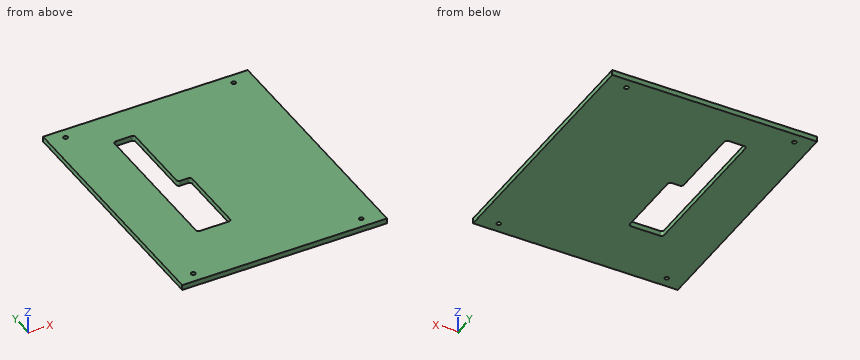
from build123d import *

# Parameters (mm, degrees)
ESQUISSE1_W        = 195
ESQUISSE1_H        = 240
ESQUISSE1_R        = 2.05
ESQUISSE1_W_2      = 32.5
ESQUISSE1_H_2      = 145
ESQUISSE1_W_3      = 12.5
ESQUISSE1_H_3      = 75
BOSS_EXTRU_1_DEPTH = 5
CONG_1_R           = 2.5


with BuildPart() as part:
    # Esquisse1 → Boss.-Extru.1 (new body)
    # profile 1 of 2: a face of its own
    with BuildSketch(Plane.XY):
        with Locations((-22.5, 0)):
            Rectangle(ESQUISSE1_W, ESQUISSE1_H)
        with Locations((56, -110)):
            Circle(ESQUISSE1_R, mode=Mode.SUBTRACT)
        with Locations((56, 110)):
            Circle(ESQUISSE1_R, mode=Mode.SUBTRACT)
        with Locations((-104, 110)):
            Circle(ESQUISSE1_R, mode=Mode.SUBTRACT)
        with Locations((-104, -110)):
            Circle(ESQUISSE1_R, mode=Mode.SUBTRACT)
        with Locations((-56.25, 12.5)):
            Rectangle(ESQUISSE1_W_2, ESQUISSE1_H_2, mode=Mode.SUBTRACT)
    # profile 2 of 2: a face of its own
    with BuildSketch(Plane.XY):
        with Locations((-46.25, 47.5)):
            Rectangle(ESQUISSE1_W_3, ESQUISSE1_H_3)
    extrude(amount=BOSS_EXTRU_1_DEPTH)

    # Congé1
    cong_1_edges = [part.edges().sort_by_distance(p)[0] for p in [
        (-72.5, 85, 2.5),
        (-72.5, -60, 2.5),
        (-40, -60, 2.5),
        (-40, 10, 2.5),
        (-52.5, 10, 2.5),
        (-52.5, 85, 2.5),
    ]]
    fillet(cong_1_edges, radius=CONG_1_R)


solid = part.part
Verification items for the finished model (mm, model axes). Coordinates: 2 decimals unless noted, no trailing zeros. Order: outer loops, then holes, each group sorted by start corner. A loop starts at its lowest first (then second) coordinate and runs counter-clockwise, first axis right, second up. Notation, with made-up numbers: M 70,15 L 80,15 A18 cw 80,21 Z; hole C -8,67.25 d1. An arc over 180 degrees is marked long. Write each question's results on one line, items separated by ' | '.
1) Section check B-B on z = 0.95. Record the cut outline in (x, y), plus the area to 3 significant figures.
Solved:
outline: M -120,-120 L 75,-120 L 75,120 L -120,120 Z; hole C -104,-110 d4.1; hole C -104,110 d4.1; hole M -72.5,-57.5 A2.5 ccw -70,-60 L -42.5,-60 A2.5 ccw -40,-57.5 L -40,7.5 A2.5 ccw -42.5,10 L -50,10 A2.5 cw -52.5,12.5 L -52.5,82.5 A2.5 ccw -55,85 L -70,85 A2.5 ccw -72.5,82.5 Z; hole C 56,-110 d4.1; hole C 56,110 d4.1 | area: 43,000 mm²
2) Section check A-A on y = 74.5. Record the cut outline in (x, z).
Solved:
outline: M -120,0 L -72.5,0 L -72.5,5 L -120,5 Z; M -52.5,0 L 75,0 L 75,5 L -52.5,5 Z
3) Scan lines: line 1 along Y through (x, z) = (-104, 2.5); line 2 along Y through (x, z) = (-49.5, 2.65); line 3 along X through (y, z) = (72.5, 2.25). Record each from-to range of solid material in increasing order. Write a range as [from, to].
Solved:
line 1: y = [-120, -112.05], [-107.95, 107.95], [112.05, 120] | line 2: y = [-120, -60], [10, 120] | line 3: x = [-120, -72.5], [-52.5, 75]
4) Gauge pin test, flat end, axial feed: pin 1 Ø5.5 at (x, y) = (56, 110) entering from +Z. Record the tip position at first contact, or that the pin passes through.
Solved:
pin 1: stops at z = 5
